from build123d import *

# Parameters (mm, degrees)
ESQUISSE1_R             = 4
EXTRUSION1_DEPTH        = 10
EXTRUSION1_DEPTH_BACK   = 3
ESQUISSE2_R             = 5
EXTRUSION2_DEPTH        = 3
ENL_V_MAT_EXTRU_1_DEPTH = 3
ESQUISSE4_R             = 2.5
ENL_V_MAT_EXTRU_2_DEPTH = 14


with BuildPart() as part:
    # Esquisse1 → Extrusion1 (new body, two sides)
    with BuildSketch(Plane(origin=(0, 0, 0), x_dir=(0, 0, -1), z_dir=(1, 0, 0))) as extrusion1_sk:
        Circle(ESQUISSE1_R)
    extrude(amount=EXTRUSION1_DEPTH)
    extrude(extrusion1_sk.sketch, amount=-EXTRUSION1_DEPTH_BACK)

    # Esquisse2 → Extrusion2 (add)
    with BuildSketch(Plane(origin=(0, 0, 0), x_dir=(0, 0, -1), z_dir=(1, 0, 0))):
        Circle(ESQUISSE2_R)
    extrude(amount=-EXTRUSION2_DEPTH)

    # Esquisse3 → Enlèv. mat.-Extru.1 (cut)
    with BuildSketch(Plane.ZY.offset(3)):
        Polygon((0, 2.886751346), (-2.5, 1.443375673), (-2.5, -1.443375673), (0, -2.886751346), (2.5, -1.443375673), (2.5, 1.443375673), align=None)
    extrude(amount=-ENL_V_MAT_EXTRU_1_DEPTH, mode=Mode.SUBTRACT)

    # Esquisse4 → Enlèv. mat.-Extru.2 (cut, through all)
    with BuildSketch(Plane(origin=(10, 0, 0), x_dir=(0, 0, -1), z_dir=(1, 0, 0))):
        Circle(ESQUISSE4_R)
    extrude(amount=-ENL_V_MAT_EXTRU_2_DEPTH, mode=Mode.SUBTRACT)


solid = part.part
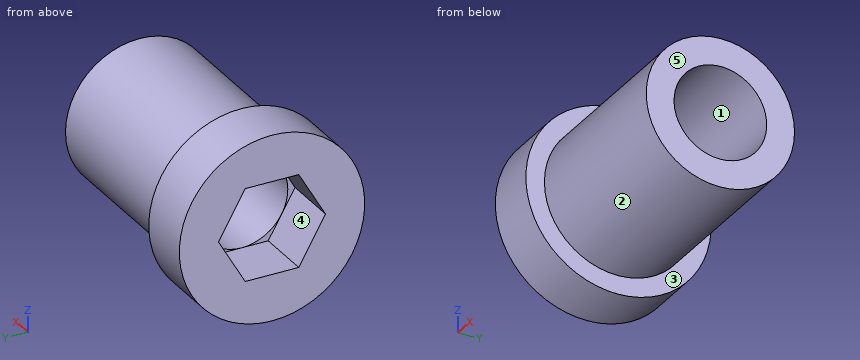
The model under review builds one solid part; all positions refer to its coordinate system, in mm. Face numbers are marked on the shaded views. A direction names the side the tool comes from. Coordinates: 2 decimals unless noted, no trailing zeros. Order: outer loops, then holes, each group sorted by start corner. A loop starts at its lowest first (then second) coordinate and runs counter-clockwise, first axis right, second up. Notation, with made-up numbers: (-30, 67.25) -> (25, 67.25) arc R25 ccw to (25, 90.25) -> close; hole circle Ø10 at (-25.5, 82). An arc over 180 degrees is marked (long way). Answer in a Markdown table with one row per item.
(1) Insertion check: pin 1 (1.5 mm diameter, centred on x = 6.5, z = -0.5, fed in from +Y); pin 2 (1.4 mm diameter, centred on x = -1, y = 0.5, fed in from -Z); pin 3 (3 mm diameter, centred on x = 0.5, y = -4, fed in from -Z); pin 4 (4 mm diameter, centred on x = 2.5, y = -1.5, fed in from +Z). Each pin has a flat end and moves straight along its axis. Give the tip position at first contact, or say it passes through.
Answers:
| item | result |
|---|---|
| pin 1 | y = 4 |
| pin 2 | z = -5 |
| pin 3 | z = -4.28 |
| pin 4 | z = 4 |
(2) Machinability: for the marked faces 4 and 5, which of the approach directions +Z, -Z, +X, -X, +Y, -Y give a long, thin tool a straight path to every point of the face, cutting with its end or side? Answer none if there is none.
Answers:
| item | result |
|---|---|
| face 4 | -X |
| face 5 | +Z, -Z, +X, +Y, -Y |
(3) Wall thickness on line 1 along Y through (x, z) = (3.25, 0); line 2 along Y through (x, z) = (-1.75, 1.5); line 3 along Y through (x, z) = (-0.25, 3): over which ranges is each line inside the solid? List them lowest first.
Answers:
| item | result |
|---|---|
| line 1 | -4 to -2.5, 2.5 to 4 |
| line 2 | -4.77 to -2.02, 2.02 to 4.77 |
| line 3 | -4 to 4 |
(4) Consider section B-B (y = 0.5). Write out the cut boundary in (x, z).
Answers:
| item | result |
|---|---|
| outline | (-3, -4.97) -> (0, -4.97) -> (0, -3.97) -> (10, -3.97) -> (10, -2.45) -> (0, -2.45) -> (0, -2.5) -> (-3, -2.5) -> close; (-3, 2.5) -> (0, 2.5) -> (0, 2.45) -> (10, 2.45) -> (10, 3.97) -> (0, 3.97) -> (0, 4.97) -> (-3, 4.97) -> close |
(5) Consider section A-A (x = -1). Write out the cut boundary in (y, z).
Answers:
| item | result |
|---|---|
| outline | circle Ø10 at (0, 0); hole (-2.89, 0) -> (-1.44, -2.5) -> (1.44, -2.5) -> (2.89, 0) -> (1.44, 2.5) -> (-1.44, 2.5) -> close |
(6) Consider section D-D (z = -2.75). Write out the cut boundary in (x, y).
Answers:
| item | result |
|---|---|
| outline | (-3, -4.18) -> (0, -4.18) -> (0, -2.9) -> (10, -2.9) -> (10, 2.9) -> (0, 2.9) -> (0, 4.18) -> (-3, 4.18) -> close |
(7) The part is to be moulded in two halves that separate along Z. For the marked faces 1, 2 and 3, say which applies: +Z half, -Z half, draft (parallel to the pull), parting line (faces both ways), or undercut.
Answers:
| item | result |
|---|---|
| face 1 | undercut |
| face 2 | parting line |
| face 3 | draft |
